Build history of the part. All positions in model axes, mm. A direction names the side the tool comes from. Give positions to 0.01 mm unless a question says otherwise; leave off trailing zeros. Order: outer loops, then holes, each group sorted by start corner. A loop starts at its lowest first (then second) coordinate and runs counter-clockwise, first axis right, second up. Notation, with made-up numbers: (4, -29.5) - (15, -29.5) arc R20 ccw to (15, 2.5) - close; hole circle Ø4 at (21, 15.25). An arc over 180 degrees is marked (long way). One line per item, written item: value.
```python
from build123d import *

# Parameters (mm, degrees)
SKETCH1_W           = 30
SKETCH1_H           = 13
BOSS_EXTRUDE1_DEPTH = 0.6
BOSS_EXTRUDE2_DEPTH = 1
FILLET1_R           = 2
SKETCH3_R           = 1.75
CUT_EXTRUDE1_DEPTH  = 2.6


with BuildPart() as part:
    # Sketch1 → Boss-Extrude1 (new body)
    with BuildSketch(Plane(origin=(0, 0, 0), x_dir=(1, 0, 0), z_dir=(0, 1, 0))):
        Rectangle(SKETCH1_W, SKETCH1_H)
    extrude(amount=BOSS_EXTRUDE1_DEPTH)

    # Sketch2 → Boss-Extrude2 (add)
    with BuildSketch(Plane(origin=(0, 0.6, 0), x_dir=(1, 0, 0), z_dir=(0, 1, 0))):
        Polygon((-13, 4.5), (13, 4.5), (13, -6.5), (15, -6.5), (15, 6.5), (-15, 6.5), (-15, -6.5), (-13, -6.5), align=None)
    extrude(amount=BOSS_EXTRUDE2_DEPTH)

    # Fillet1
    fillet1_edges = [part.edges().sort_by_distance(p)[0] for p in [
        (-15, 0.8, 6.5),
        (15, 0.8, 6.5),
        (15, 0.8, -6.5),
        (-15, 0.8, -6.5),
    ]]
    fillet(fillet1_edges, radius=FILLET1_R)

    # Sketch3 → Cut-Extrude1 (cut, through all)
    with BuildSketch(Plane.XZ):
        with Locations((-5, 1.7)):
            Circle(SKETCH3_R)
        with Locations((5, 1.7)):
            Circle(SKETCH3_R)
    extrude(amount=-CUT_EXTRUDE1_DEPTH, mode=Mode.SUBTRACT)


solid = part.part
```
(1) Pin check, flat tips, straight feed: P1, Ø0.5, axis at x = 0.5, y = 1, coming from the +Z side; P2, Ø4, axis at x = 5, z = 1.7, coming from the +Y side. Stop position of each tip, or through.
Completed:
P1: z = -4.5
P2: y = 0.6
(2) 3-axis set-ups, long thin cutter, end or side, ignore diameter. For faces 1 (the face through (-13, 1, 1)), 2 (the face through (0, 1, -6.5)): which of +Z, -Z, +X, -X, +Y, -Y reach the whole face in a straight line?
Completed:
face 1: +Z, +Y
face 2: -Z, +X, -X, +Y, -Y
(3) Slice it at A-A, the plane z = 2.75. Give the cut face in (x, y).
Completed:
outline: (-15, 0) - (-6.4, 0) - (-6.4, 0.6) - (-13, 0.6) - (-13, 1.6) - (-15, 1.6) - close; (-3.6, 0) - (3.6, 0) - (3.6, 0.6) - (-3.6, 0.6) - close; (6.4, 0) - (15, 0) - (15, 1.6) - (13, 1.6) - (13, 0.6) - (6.4, 0.6) - close
(4) Slice it at C-C, the plane x = 5. Give the cut face in (y, z), and give its area (3 significant figures).
Completed:
outline: (0, -6.5) - (1.6, -6.5) - (1.6, -4.5) - (0.6, -4.5) - (0.6, -0.05) - (0, -0.05) - close; (0, 3.45) - (0.6, 3.45) - (0.6, 6.5) - (0, 6.5) - close
area: 7.70 mm²
(5) Drill centre lines: line 1 (Z direction, x = 5, y = 0.25); line 2 (X direction, y = 1.2, z = 1); line 3 (Y direction, x = 1, z = 2.25). Where is each one in solid material? Low to high.
Completed:
line 1: -6.5 to -0.05, 3.45 to 6.5
line 2: -15 to -13, 13 to 15
line 3: 0 to 0.6
(6) Slice it at D-D, the plane z = -1.25. Give the cut face in (x, y).
Completed:
outline: (-15, 0) - (15, 0) - (15, 1.6) - (13, 1.6) - (13, 0.6) - (-13, 0.6) - (-13, 1.6) - (-15, 1.6) - close
(7) Slice it at B-B, the plane y = 0.3. Give the cut face in (x, z), and give its area (3 significant figures).
Completed:
outline: (-15, -4.5) arc R2 ccw to (-13, -6.5) - (13, -6.5) arc R2 ccw to (15, -4.5) - (15, 4.5) arc R2 ccw to (13, 6.5) - (-13, 6.5) arc R2 ccw to (-15, 4.5) - close; hole circle Ø3.5 at (-5, 1.7); hole circle Ø3.5 at (5, 1.7)
area: 367 mm²
(8) Pull direction X, two halves, no side cores. Call faces 3 (the face through (0, 0.6, 1)), 4 (the face through (-14.43, 0.79, 5.9)), 5 (the face through (14.4, 0.81, -5.93)): +X half, -X half, draft (parallel to the pull), parting line (faces both ways), or undercut.
Completed:
face 3: undercut
face 4: -X half
face 5: +X half
